Verification items for the finished model (mm, model axes). Face numbers are marked on the shaded views. Coordinates: 2 decimals unless noted, no trailing zeros. Write each loop counter-clockwise with the first axis right and the second up, starting at its lowest first coordinate (ties: lowest second). Pieces come first, ordered by that corner, then holes. Notation, with made-up numbers: (87.5, -15.5) -> (112.5, -15.5) arc R28 ccw to (112.5, 6.5) -> close; hole circle Ø9 at (-24.75, 53). An arc over 180 degrees is marked (long way). Use CSV: the item, a comma, the result in double quotes.
```python
from build123d import *

# Parameters (mm, degrees)
EXTRUDE009_DEPTH = 150
EXTRUDE008_DEPTH = 667


with BuildPart() as extrude009:
    # Sketch010 (on Face2 of Extrude008) → Extrude009 (new body)
    with BuildSketch(Plane.XY.offset(4500)):
        Polygon((500, 667), (575, 592), (575, 667), align=None)
    extrude(amount=-EXTRUDE009_DEPTH)


with BuildPart() as compound008:
    # Mirror008: instance of Extrude009
    add(extrude009.part.mirror(Plane(origin=(300, 0, 0), x_dir=(1, 0, 0), z_dir=(0, 1, 0))))

    # Compound008: union Extrude009
    add(extrude009.part)


with BuildPart() as cut002:
    # ChannelSteel002 → Extrude008 (new body, symmetric)
    with BuildSketch(Plane(origin=(521.664812, 0, 4425), x_dir=(1, 0, 0), z_dir=(0, 1, 0))):
        with BuildLine():
            Line((-21.664812, 75), (-21.664812, -75))
            Line((-21.664812, -75), (53.335188, -75))
            Line((53.335188, -75), (53.335188, -73.913145))
            ThreePointArc((53.335188, -73.913145), (51.364768, -68.846219), (46.488856, -66.441685))
            Line((46.488856, -66.441685), (3.642524, -62.693117))
            ThreePointArc((3.642524, -62.693117), (-7.792334, -58.760281), (-12.664812, -47.693117))
            Line((-12.664812, -47.693117), (-12.664812, 47.693117))
            ThreePointArc((-12.664812, 47.693117), (-7.792334, 58.760281), (3.642524, 62.693117))
            Line((3.642524, 62.693117), (46.488856, 66.441685))
            ThreePointArc((46.488856, 66.441685), (51.364768, 68.846219), (53.335188, 73.913145))
            Line((53.335188, 73.913145), (53.335188, 75))
            Line((53.335188, 75), (-21.664812, 75))
        make_face()
    extrude(amount=EXTRUDE008_DEPTH, both=True)

    # Cut002: cut Compound008
    add(compound008.part, mode=Mode.SUBTRACT)


with BuildPart() as cut002_mirrored:
    # Mirror009: instance of Cut002
    add(cut002.part.mirror(Plane(origin=(0, -600, 0), x_dir=(0, -1, 0), z_dir=(1, 0, 0))))


solid = cut002_mirrored.part
```
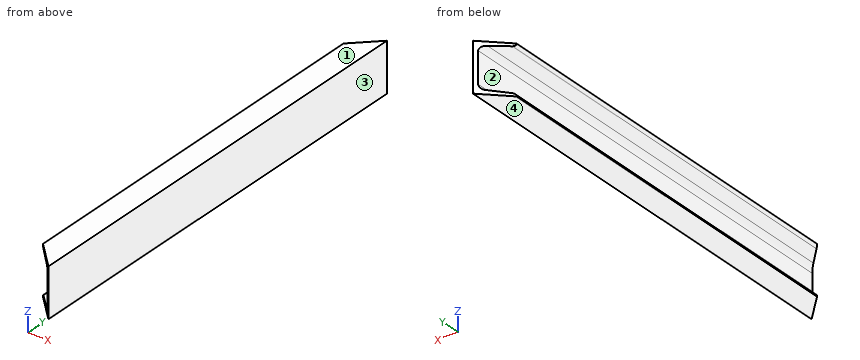
1) Gauge pin test, flat end, axial feed: pin 1 (3 mm diameter, centred on y = -234, z = 4389, fed in from -X). Record the tip position at first contact, or that the pin passes through.
Return value:
pin 1,"x = -509"
2) Scan lines: L1, parallel to Z at x = -524, y = 234; L2, parallel to X at y = 3, z = 4461.5; L3, parallel to Z at x = -518.5, y = -201. Record each from-to range of solid material in increasing order.
Return value:
L1,"4350 to 4362.26, 4487.74 to 4500"
L2,"-509 to -500"
L3,"4350 to 4363.33, 4486.67 to 4500"
3) Cross-section at A-A (y = 187.5). Record the boundary of the cut face in (x, z).
Return value:
outline,"(-575, 4350) -> (-500, 4350) -> (-500, 4500) -> (-575, 4500) -> (-575, 4498.91) arc R7.5 ccw to (-568.15, 4491.44) -> (-525.31, 4487.69) arc R15.08 cw to (-509, 4472.69) -> (-509, 4377.31) arc R15.08 cw to (-525.31, 4362.31) -> (-568.15, 4358.56) arc R7.5 ccw to (-575, 4351.09) -> close"
4) Cross-section at C-C (z = 4454.5). Record the boundary of the cut face in (x, y), plus the area to 3 significant figures.
Return value:
outline,"(-509, -658) -> (-500, -667) -> (-500, 667) -> (-509, 658) -> close"
area,"11,900 mm2"
5) Cross-section at B-B (x = -551). Record the boundary of the cut face in (y, z), plus the area to 3 significant figures.
Return value:
outline,"(-616, 4350) -> (616, 4350) -> (616, 4360.06) -> (-616, 4360.06) -> close; (-616, 4489.94) -> (616, 4489.94) -> (616, 4500) -> (-616, 4500) -> close"
area,"24,800 mm2"
6) Mould release check, pull along Z, two halves, no side actions. Record for the marked faces 1, 2, 3 and 4: released by +Z, released by -Z, zero draft, split by the parting line, or undercut.
Return value:
face 1,"released by +Z"
face 2,"undercut"
face 3,"zero draft"
face 4,"released by -Z"
